```python
from build123d import *

# Parameters (mm, degrees)
SKETCH1_W           = 12.7
SKETCH1_H           = 12.7
BOSS_EXTRUDE1_DEPTH = 2.54
FILLET1_R           = 0.635
SHELL1_START        = 0.635
SHELL1_OUTLINE_W    = 1.905
SHELL1_OUTLINE_H    = 11.43
SHELL1_DEPTH        = 11.43
SKETCH2_R           = 2.54
BOSS_EXTRUDE2_DEPTH = 1.905
BOSS_EXTRUDE3_DEPTH = 0.00254


# Read off the part's stored shape, not the designer's step: Shell1
with BuildPart() as part:
    # Sketch1 → Boss-Extrude1 (new body)
    with BuildSketch(Plane(origin=(0, 0, 0), x_dir=(1, 0, 0), z_dir=(0, 1, 0))):
        with Locations((6.35, 6.35)):
            Rectangle(SKETCH1_W, SKETCH1_H)
    extrude(amount=BOSS_EXTRUDE1_DEPTH)

    # Fillet1
    fillet1_edges = [part.edges().sort_by_distance(p)[0] for p in [
        (0, 1.27, -12.7),
        (12.7, 1.27, -12.7),
        (12.7, 1.27, 0),
        (0, 1.27, 0),
    ]]
    fillet(fillet1_edges, radius=FILLET1_R)

    # Shell1 outline → Shell1 (cut)
    with BuildSketch(Plane.YZ.offset(SHELL1_START)):
        with Locations((0.9525, -6.35)):
            Rectangle(SHELL1_OUTLINE_W, SHELL1_OUTLINE_H)
    extrude(amount=SHELL1_DEPTH, mode=Mode.SUBTRACT)

    # Sketch2 → Boss-Extrude2 (add)
    with BuildSketch(Plane(origin=(0, 1.905, 0), x_dir=(-1, 0, 0), z_dir=(0, -1, 0))):
        with Locations(Location((-6.35, 6.35, 0), (0, 0, 270))):
            Circle(SKETCH2_R)
    extrude(amount=BOSS_EXTRUDE2_DEPTH)

    # Sketch3 → Boss-Extrude3 (add)
    with BuildSketch(Plane(origin=(0, 2.54, 0), x_dir=(1, 0, 0), z_dir=(0, 1, 0))):
        Polygon((5.334325641, 8.001), (7.247466667, 8.001), (6.110267147, 5.395871795), (7.16605641, 5.395871795), (7.16605641, 4.826), (5.252915385, 4.826), (6.390750921, 7.431128205), (5.334325641, 7.431128205), align=None)
    extrude(amount=BOSS_EXTRUDE3_DEPTH)


solid = part.part
```
Read the model definition and answer for the solid it produces. Units are mm, in the model's axes. A direction names the side the tool comes from. Round coordinates to 2 decimals unless told otherwise and drop trailing zeros. Loops run counter-clockwise (first coordinate to the right, second up) from the corner with the lowest first, then second, coordinate; pieces in that order, holes last. Notation, with made-up numbers: (19.5, -26) -> (75.5, -26) arc R9 ccw to (75.5, -20) -> close; hole circle Ø5 at (79.5, 8.5). An arc over 180 degrees is marked (long way). One line per item, written item: value.
1) For faces 1 (the face through (6, 0, -6)), 2 (the face through (6, 1, -12.065)), determine the directions among +Z, -Z, +X, -X, +Y, -Y from which every point of the face is accessible in a straight line to the end or side of a thin tool.
Answer list:
face 1: +Z, -Z, +X, -X, -Y
face 2: -Y
2) A cutting plane is placed at B-B (z = -11). Determine the outline of the cut face in (x, y) (3 decimals).
Answer list:
outline: (0, 0) -> (0.635, 0) -> (0.635, 1.905) -> (12.065, 1.905) -> (12.065, 0) -> (12.7, 0) -> (12.7, 2.54) -> (0, 2.54) -> close
3) A flat-ended cylindrical pin translates along its axis: P1, Ø2, axis at x = 9.5, z = -1.5, coming from the +Y side. Find the tip coordinate at first contact, or state that the pin passes through.
Answer list:
P1: stops at y = 2.54
4) A cutting plane is placed at A-A (y = 1). Determine the outline of the cut face in (x, z) (3 decimals), and give its area (3 significant figures).
Answer list:
outline: (0, -12.065) arc R0.635 ccw to (0.635, -12.7) -> (12.065, -12.7) arc R0.635 ccw to (12.7, -12.065) -> (12.7, -0.635) arc R0.635 ccw to (12.065, 0) -> (0.635, 0) arc R0.635 ccw to (0, -0.635) -> close; circle Ø5.08 at (6.35, -6.35); hole (0.635, -12.065) -> (12.065, -12.065) -> (12.065, -0.635) -> (0.635, -0.635) -> close
area: 50.6 mm²
5) Consider L1, parallel to X at y = 1.1, z = -9.75 (3 decimals); L2, parallel to Z at x = 3.5, y = 0.45 (3 decimals); L3, parallel to Z at x = 6.75, y = 0.8 (3 decimals). Determine where each line is inside the solid, lowest interval first. Write a range as [from, to].
Answer list:
L1: x = [0, 0.635], [12.065, 12.7]
L2: z = [-12.7, -12.065], [-0.635, 0]
L3: z = [-12.7, -12.065], [-8.858, -3.842], [-0.635, 0]
6) A cutting plane is placed at C-C (x = 3). Determine the outline of the cut face in (y, z) (3 decimals).
Answer list:
outline: (0, -12.7) -> (2.54, -12.7) -> (2.54, 0) -> (0, 0) -> (0, -0.635) -> (1.905, -0.635) -> (1.905, -12.065) -> (0, -12.065) -> close
7) The mould has two halves that part along X. Classify faces 3 (the face through (6, 1, -0.635)), 4 (the face through (0, 1, -6)), 5 (the face through (12.065, 1, -6)), 6 (the face through (6, 1, -12.7)): pulls with the +X half, pulls with the -X half, needs draft (parallel to the pull), parting line crosses it, or undercut.
Answer list:
face 3: undercut
face 4: pulls with the -X half
face 5: undercut
face 6: needs draft
